The listing builds one solid part. Answer for the finished solid, in the listing's coordinates (mm). Face numbers are marked on the shaded views. Coordinates: 2 decimals unless noted, no trailing zeros. Order: outer loops, then holes, each group sorted by start corner. A loop starts at its lowest first (then second) coordinate and runs counter-clockwise, first axis right, second up. Notation, with made-up numbers: (15, -6.75) -> (32, -6.75) arc R24 cw to (32, 16.25) -> close; hole circle Ø4 at (52.5, -3.75). An arc over 180 degrees is marked (long way). Write item = value, one per line.
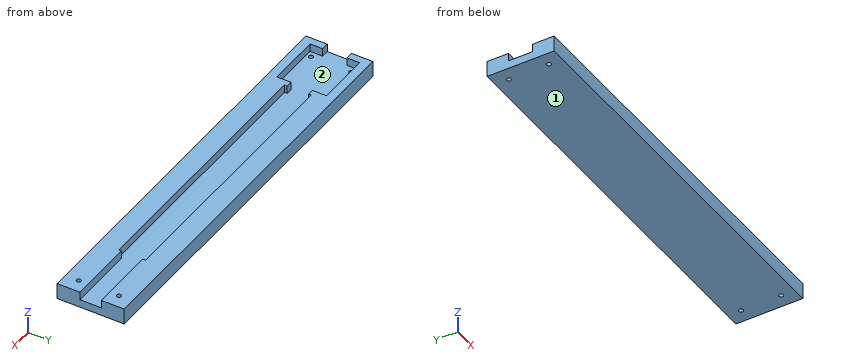
from build123d import *

# Parameters (mm, degrees)
SKETCH_W              = 150
SKETCH_H              = 25
PAD_DEPTH             = 3
PAD001_DEPTH          = 3
SKETCH003_R           = 0.825
POCKET_DEPTH          = 313.375769
POLARPATTERN_COUNT    = 2
POLARPATTERN001_COUNT = 2
POLARPATTERN002_COUNT = 2


with BuildPart() as part:
    # Sketch → Pad (new body)
    with BuildSketch(Plane.XY):
        Rectangle(SKETCH_W, SKETCH_H)
    extrude(amount=PAD_DEPTH)

    # Sketch001 (on Face6 of Pad) → Pad001 (join)
    with BuildSketch(Plane.XY.offset(3)):
        Polygon((-75, 12.5), (75, 12.5), (75, 4), (50, 4), (50, 5), (-50, 5), (-50, 4), (-52.25, 4), (-52.25, 9.2), (-72.25, 9.2), (-72.25, 4.5), (-75, 4.5), align=None)
        Polygon((-75, -12.5), (75, -12.5), (75, -4), (50, -4), (50, -5), (-50, -5), (-50, -4), (-52.25, -4), (-52.25, -9.2), (-72.25, -9.2), (-72.25, -4.5), (-75, -4.5), align=None)
    extrude(amount=PAD001_DEPTH)

    # Sketch003 → Pocket (cut, through all)
    with BuildSketch(Plane.XY.offset(9)):
        with Locations((-70, 7.5)):
            Circle(SKETCH003_R)
    pocket = extrude(amount=-POCKET_DEPTH, mode=Mode.SUBTRACT)

    # PolarPattern: Pocket ×2 about axis
    polarpattern_axis = Axis((0, 0, 0), (0, 1, 0))
    for i in range(1, POLARPATTERN_COUNT):
        add(pocket.rotate(polarpattern_axis, i * 360 / POLARPATTERN_COUNT), mode=Mode.SUBTRACT)

    # PolarPattern001: Pocket ×2 about axis
    polarpattern001_axis = Axis((0, 0, 0), (1, 0, 0))
    for i in range(1, POLARPATTERN001_COUNT):
        add(pocket.rotate(polarpattern001_axis, i * 360 / POLARPATTERN001_COUNT), mode=Mode.SUBTRACT)

    # PolarPattern002: Pocket ×2 about axis
    polarpattern002_axis = Axis((0, 0, 9), (0, 0, 1))
    for i in range(1, POLARPATTERN002_COUNT):
        add(pocket.rotate(polarpattern002_axis, i * 360 / POLARPATTERN002_COUNT), mode=Mode.SUBTRACT)


solid = part.part
Q1. Each of these flat-tipped pins is pushed along its axis until it touches: pin 1 Ø1.5 at (x, y) = (-70, -7.5) entering from +Z; pin 2 Ø2.5 at (x, y) = (-70, 7.5) entering from +Z. Where does it stop, or does it pass through?
The answers:
pin_1 = through
pin_2 = 3
Q2. Find the intervals of material crossed by line 1 along X through (y, z) = (-7.5, 1.9) (3 decimals); line 2 along X through (y, z) = (-7.5, 3.55) (3 decimals); line 3 along Y through (x, z) = (70, 2.05) (3 decimals), in increasing order.
The answers:
line_1 = -75 to -70.825, -69.175 to 69.175, 70.825 to 75
line_2 = -75 to -72.25, -52.25 to 69.175, 70.825 to 75
line_3 = -12.5 to -8.325, -6.675 to 6.675, 8.325 to 12.5
Q3. The mould has two halves that part along Y. Classify the marked faces 1 and 2: released by +Y, released by -Y, zero draft, split by the parting line, or undercut.
The answers:
face_1 = zero draft
face_2 = undercut
Q4. Section A-A, the plane z = 4.4 is taken. Give the vertices of the cut face in (x, y) (3 decimals), plus the area to 3 significant figures.
The answers:
outline = (-75, -12.5) -> (75, -12.5) -> (75, -4) -> (50, -4) -> (50, -5) -> (-50, -5) -> (-50, -4) -> (-52.25, -4) -> (-52.25, -9.2) -> (-72.25, -9.2) -> (-72.25, -4.5) -> (-75, -4.5) -> close; (-75, 4.5) -> (-72.25, 4.5) -> (-72.25, 9.2) -> (-52.25, 9.2) -> (-52.25, 4) -> (-50, 4) -> (-50, 5) -> (50, 5) -> (50, 4) -> (75, 4) -> (75, 12.5) -> (-75, 12.5) -> close; hole circle Ø1.65 at (70, -7.5); hole circle Ø1.65 at (70, 7.5)
area = 2,130 mm2
Q5. Section B-B, the plane x = 15 is taken. Give the vertices of the cut face in (y, z), plus the area to 3 significant figures.
The answers:
outline = (-12.5, 0) -> (12.5, 0) -> (12.5, 6) -> (5, 6) -> (5, 3) -> (-5, 3) -> (-5, 6) -> (-12.5, 6) -> close
area = 120 mm2
